Check sheet for the modelled part. Datum: model origin and axes. Units: mm. Face numbers are marked on the shaded views. Round coordinates to 2 decimals unless told otherwise and drop trailing zeros. Loops run counter-clockwise (first coordinate to the right, second up) from the corner with the lowest first, then second, coordinate; pieces in that order, holes last. Notation, with made-up numbers: (27.5, 73.5) -> (69.5, 73.5) arc R17 cw to (69.5, 93.5) -> close; hole circle Ø7 at (29, 77.25). An arc over 180 degrees is marked (long way). Return JSON: item names as keys, results as strings.
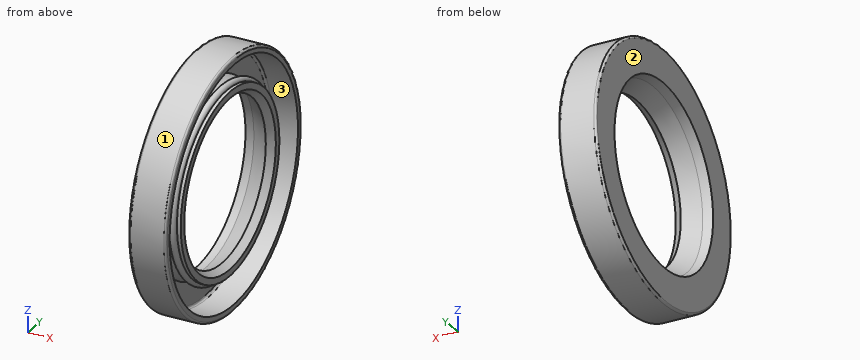
Autodesk Inventor part; units mm, degrees
ref_plane "YZ Plane" through (0, 0, 0) normal (1, 0, 0) x (0, 1, 0)
ref_plane "XZ Plane" through (0, 0, 0) normal (0, 1, 0) x (-1, 0, 0)
ref_plane "XY Plane" through (0, 0, 0) normal (0, 0, 1) x (1, 0, 0)
sketch "Эскиз1" plane through (0, 0, 0) normal (0, 0, 1) x (1, 0, 0)
  circle A0 centre (4.9, 17.1) radius 0.455
  circle A1 centre (4.9, 17.1) radius 0.7
  line L0 (6.3, 15.875) -> (6.3, 17.1)
  line L1 (0, 23.5) -> (7, 23.5)
  line L2 (7, 23.5) -> (7, 22.25)
  line L3 (7, 22.25) -> (1.75, 22.25)
  line L4 (0, 0) -> (9.5856, 0)
  line L5 (0, 23.5) -> (0, 17.1)
  line L6 (0, 17.1) -> (1.75, 16.75)
  line L7 (1.75, 16.75) -> (4.9, 15)
  line L8 (4.9, 15) -> (6.3, 15.875)
  line L9 (4.9, 15) -> (0, 15) construction
  line L10 (0, 18) -> (0, -3)
  line L11 (-1.9171, 0) -> (11.5027, 0)
  line L12 (4.2, 17.1) -> (1.75, 17.59)
  line L13 (1.75, 17.59) -> (1.75, 22.25)
  line L14 (6.3, 17.1) -> (5.6, 17.1)
  dimension "d0" = 47
  dimension "d1" = 31.75
  dimension "d2" = 1.25
  dimension "d3" = 0.91
  dimension "d4" = 1.4
  dimension "d5" = 30
  dimension "d6" = 33.5
  dimension "d7" = 34.2
  dimension "d8" = 4.9
  dimension "d9" = 6.3
  dimension "d10" = 7
  dimension "d12" = 1.75
revolve "Базовый элемент" add sketch "Эскиз1" angle 360 about axis through (0, 0, 0) along (1, 0, 0) contours L14 L0 L8 L7 L6 L5 L1 L2 L3 L13 L12 A1
revolve "Пружинные1" add sketch "Эскиз1" angle 360 about axis through (0, 0, 0) along (1, 0, 0) contours A0 | A1
fillet "Сопряжение1" radius 0.4 3 edges at (7, -23.5, 0) (1.75, -22.25, 0) (0, -23.5, 0)
equation "\"d0\" = SD2"
equation "\"d1\" = ABDM"
equation "\"d3\" = SPDI"
equation "\"d4\" = SPDA"
equation "\"d5\" = NND"
equation "\"d6\" = TKDM"
equation "\"d7\" = HLDM"
equation "\"d8\" = SPDST"
equation "\"d9\" = SDI"
equation "\"d10\" = SWDT"
equation "\"d12\" = SD"
equation "\"d11\" = RR"
equation "\"SD2\" = 47"
equation "\"SWDT\" = 7"
equation "\"RR\" = 0.4"
equation "\"SD\" = 1.75"
equation "\"NND\" = 30"
equation "\"SPDA\" = 1.4"
equation "\"SPDI\" = 0.91"
equation "\"TKDM\" = 33.5"
equation "\"HLDM\" = 34.2"
equation "\"ABDM\" = 31.75"
equation "\"SDI\" = 6.3"
equation "\"SPDST\" = 4.9"
equation "\"LAB\" = 0.35"
properties part number "Манжет 1-30x47x7 ГОСТ 8752-79" material "Резина"
Q1. Draft check along Y on the marked faces 1, 2 and 3. Enter one of: released by +Y, released by -Y, zero draft, split by the parting line, or undercut.
Results list:
{"face 1": "split by the parting line", "face 2": "zero draft", "face 3": "undercut"}
Q2. Section check C-C (x = 1). Record the boundary of the cut face in (y, z).
Results list:
{"outline": "circle Ø47 at (0, 0); hole circle Ø33.8 at (0, 0)"}
Q3. Material ranges on line 1 (Z direction, x = 4.3, y = 0); line 2 (Z direction, x = 3.4, y = 0); line 3 (Y direction, x = 6.25, z = 4), recorded low to high.
Results list:
{"line 1": "-23.5 to -22.25, -17.46 to -15.33, 15.33 to 17.46, 22.25 to 23.5", "line 2": "-23.5 to -22.25, -17.26 to -15.83, 15.83 to 17.26, 22.25 to 23.5", "line 3": "-23.16 to -21.89, -16.63 to -15.33, 15.33 to 16.63, 21.89 to 23.16"}
Q4. Go/stop test with flat-tipped pins: pin 1 (3 mm diameter, centred on x = 5.5, y = 10, fed in from -Z); pin 2 (4 mm diameter, centred on x = 1.5, y = -17, fed in from +Z); pin 3 (2 mm diameter, centred on x = 5, y = -2.5, fed in from -Z). Record where each tip stops, or that it passes through.
Results list:
{"pin 1": "z = -21.91", "pin 2": "z = 18.09", "pin 3": "z = -23.45"}
